```python
from build123d import *

# Parameters (mm, degrees)
BOSS_EXTRU_1_DEPTH      = 3
ESQUISSE2_R             = 3
ENL_V_MAT_EXTRU_1_DEPTH = 3
ESQUISSE3_R             = 1.5
ESQUISSE3_R_2           = 1.456745064
ESQUISSE3_R_3           = 1.425181728
ENL_V_MAT_EXTRU_2_DEPTH = 10


with BuildPart() as part:
    # Esquisse1 → Boss.-Extru.1 (new body)
    with BuildSketch(Plane.XY):
        with BuildLine():
            Line((0, 0), (250, 0))
            Line((250, 0), (250, -70))
            ThreePointArc((250, -70), (247.071067812, -77.071067812), (240, -80))
            Line((240, -80), (10, -80))
            ThreePointArc((10, -80), (2.928932188, -77.071067812), (0, -70))
            Line((0, -70), (0, 0))
        make_face()
    extrude(amount=BOSS_EXTRU_1_DEPTH)

    # Esquisse2 → Enlèv. mat.-Extru.1 (cut)
    with BuildSketch(Plane.XY.offset(3)):
        with Locations((10, -75)):
            Circle(ESQUISSE2_R)
        with Locations((240, -75)):
            Circle(ESQUISSE2_R)
        with Locations((240, -10)):
            Circle(ESQUISSE2_R)
        with Locations((10, -25)):
            Circle(ESQUISSE2_R)
    extrude(amount=-ENL_V_MAT_EXTRU_1_DEPTH, mode=Mode.SUBTRACT)

    # Esquisse3 → Enlèv. mat.-Extru.2 (cut)
    with BuildSketch(Plane.XY.offset(3)):
        with Locations((26.549426967, -34.5)):
            Circle(ESQUISSE3_R)
        with Locations((64.049426967, -34.5)):
            Circle(ESQUISSE3_R_2)
        with Locations((64.049426967, -72)):
            Circle(ESQUISSE3_R_3)
        with Locations((26.549426967, -72)):
            Circle(ESQUISSE3_R)
    extrude(amount=-ENL_V_MAT_EXTRU_2_DEPTH, mode=Mode.SUBTRACT)


solid = part.part
```
Geometry check sheet. Reference: the model listing, model coordinates, mm. Give positions to 0.01 mm unless a question says otherwise; leave off trailing zeros. Loops run counter-clockwise (first coordinate to the right, second up) from the corner with the lowest first, then second, coordinate; pieces in that order, holes last. Notation, with made-up numbers: M 34.25,-2 L 71.25,-2 A20 ccw 71.25,23 Z; hole C 8.5,6 d7. An arc over 180 degrees is marked long. Write item = value, one per line. Start each with the question number.
1. Section check A-A, the plane y = -10. Enter the section's corners in (x, z).
2. Go/stop test with a flat-tipped pin: P1, Ø4, axis at x = 64.05, y = -34.5, coming from the -Z side. Record where the tip stops, or that it passes through.
3. Draft check along Y on faces 1 (the face through (12.77, -26.15, 1.52)), 2 (the face through (3.01, -77.15, 1.48)), 3 (the face through (127, -39, 0)). Enter one of: +Y half, -Y half, draft (parallel to the pull), parting line (faces both ways), or undercut.
4. Thickness scan on probe 1 along X at (y, z) = (-74.5, 2.85). Record the ranges inside material, lowest first.
Values follow:
q1.outline = M 0,0 L 237,0 L 237,3 L 0,3 Z; M 243,0 L 250,0 L 250,3 L 243,3 Z
q2.P1 = 0
q3.face_1 = undercut
q3.face_2 = -Y half
q3.face_3 = draft
q4.probe_1 = 1.07 to 7.04, 12.96 to 237.04, 242.96 to 248.93
